from build123d import *

# Parameters (mm, degrees)
SKETCH1_W                                           = 40
SKETCH1_H                                           = 25
BOSS_EXTRUDE1_DEPTH                                 = 10
CUT_EXTRUDE2_REACH                                  = 27.617
SKETCH3_W                                           = 5
SKETCH3_H                                           = 22
F_5_0MM_DOWEL_HOLE1_D                               = 5
CBORE_FOR_M5_HEX_SOCKET_HEAD_CAP_SCREW1_D           = 5.3
CBORE_FOR_M5_HEX_SOCKET_HEAD_CAP_SCREW1_CBORE_D     = 10
CBORE_FOR_M5_HEX_SOCKET_HEAD_CAP_SCREW1_CBORE_DEPTH = 5.4


with BuildPart() as part:
    # Sketch1 → Boss-Extrude1 (new body)
    with BuildSketch(Plane(origin=(0, 0, 0), x_dir=(1, 0, 0), z_dir=(0, 1, 0))):
        Rectangle(SKETCH1_W, SKETCH1_H)
    extrude(amount=BOSS_EXTRUDE1_DEPTH)

    # Sketch3 → Cut-Extrude2 (cut, up to next)
    with BuildSketch(Plane(origin=(0, 10, 0), x_dir=(1, 0, 0), z_dir=(0, 1, 0)), mode=Mode.PRIVATE) as cut_extrude2_sk1:
        with Locations((17.5, -1.5)):
            Rectangle(SKETCH3_W, SKETCH3_H)
    cut_extrude2_tool1 = extrude(cut_extrude2_sk1.sketch, amount=-CUT_EXTRUDE2_REACH, mode=Mode.PRIVATE) & part.part
    add(cut_extrude2_tool1.solids().sort_by_distance((17.5, 10, 1.5))[0], mode=Mode.SUBTRACT)

    # Ø5.0mm Dowel Hole1 (through all)
    with Locations(Plane(origin=(0, 10, 0), x_dir=(1, 0, 0), z_dir=(0, 1, 0))):
        with Locations((-15, 6), (10, -6)):
            Hole(F_5_0MM_DOWEL_HOLE1_D / 2)

    # CBORE for M5 Hex Socket Head Cap Screw1 (through all)
    with Locations(Plane(origin=(0, 10, 0), x_dir=(1, 0, 0), z_dir=(0, 1, 0))):
        with Locations((-12.5, -5), (7.5, 5)):
            CounterBoreHole(CBORE_FOR_M5_HEX_SOCKET_HEAD_CAP_SCREW1_D / 2, CBORE_FOR_M5_HEX_SOCKET_HEAD_CAP_SCREW1_CBORE_D / 2, CBORE_FOR_M5_HEX_SOCKET_HEAD_CAP_SCREW1_CBORE_DEPTH)


solid = part.part
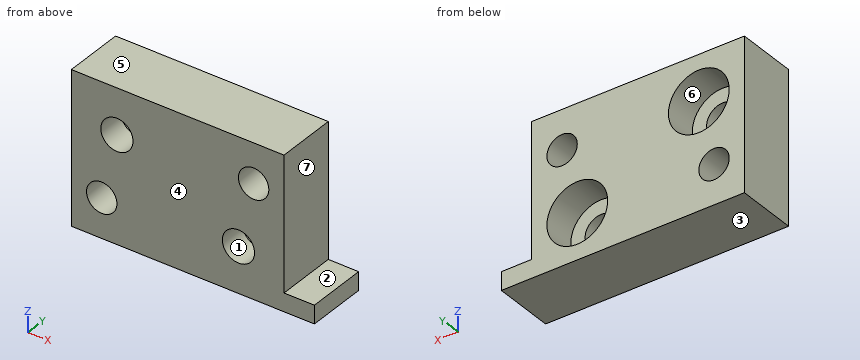
Can you work these out from the model? Positions are in its coordinate system, mm. Face numbers are marked on the shaded views. A direction names the side the tool comes from. Give positions to 0.01 mm unless a question says otherwise; leave off trailing zeros. Order: outer loops, then holes, each group sorted by start corner. A loop starts at its lowest first (then second) coordinate and runs counter-clockwise, first axis right, second up. Notation, with made-up numbers: M 0.5,11.25 L 58.5,11.25 A21 ccw 58.5,45.25 Z; hole C 32,-1 d10. An arc over 180 degrees is marked long. Use a Markdown table: item, result. Add a question column.
Item 1: We'd pull the mould along Z, two halves only. Please class the marked faces 1, 2, 3 and 4: +Z half, -Z half, draft (parallel to the pull), parting line (faces both ways), or undercut.
Item 2: Will these pins go through, and if not, where does the flat tip stop? pin 1 (1 mm diameter, centred on y = 4, z = 9.5, fed in from +X); pin 2 (4.5 mm diameter, centred on x = -15, z = -6, fed in from +Y); pin 3 (11.5 mm diameter, centred on x = 7.5, z = -5, fed in from -Y); pin 4 (4 mm diameter, centred on x = 18.5, y = 3.5, fed in from +Z).
Item 3: Suppose I cut it at C-C (x = 11). List the corners of the cut face in (y, z) for me, then the cut area to 3 significant figures.
Item 4: If I drill on L1, parallel to X at y = 8.25, z = -7; L2, parallel to X at y = 3.5, z = 10; L3, parallel to Y at x = 9, z = -9, over which ranges is the centre line in solid material (lowest first)? Write a range as [from, to].
Item 5: Suppose I cut it at D-D (x = -14.5). List the corners of the cut face in (y, z) for me, then the cut area to 3 significant figures.
Item 6: Suppose I cut it at A-A (y = 7). List the corners of the cut face in (x, z) for me, then the cut area to 3 significant figures.
Item 7: Suppose I cut it at B-B (z = 6). List the corners of the cut face in (x, y) for me.
Item 8: For the marked faces 5, 6 and 7, which set-ups out of +Z, -Z, +X, -X, +Y, -Y let a thin tool reach every point of the face, with its end or its side?
Answer sheet:
| question | item | result |
|---|---|---|
| 1 | face 1 | undercut |
| 1 | face 2 | +Z half |
| 1 | face 3 | -Z half |
| 1 | face 4 | draft |
| 2 | pin 1 | stops at x = 15 |
| 2 | pin 2 | passes through |
| 2 | pin 3 | stops at y = 0 |
| 2 | pin 4 | stops at z = -9.5 |
| 3 | outline | M 0,-12.5 L 10,-12.5 L 10,-8.57 L 4.6,-8.57 L 4.6,-1.43 L 10,-1.43 L 10,3.71 L 0,3.71 Z; M 0,8.29 L 10,8.29 L 10,12.5 L 0,12.5 Z |
| 3 | area | 166 mm² |
| 4 | L1 | x = [-20, -17.29], [-12.71, 2.92], [12.08, 15] |
| 4 | L2 | x = [-20, 15] |
| 4 | L3 | y = [0, 4.6] |
| 5 | outline | M 0,-12.5 L 10,-12.5 L 10,-8.45 L 0,-8.45 Z; M 0,-3.55 L 10,-3.55 L 10,0.42 L 4.6,0.42 L 4.6,3.26 L 0,3.26 Z; M 0,6.74 L 4.6,6.74 L 4.6,9.58 L 10,9.58 L 10,12.5 L 0,12.5 Z |
| 5 | area | 136 mm² |
| 6 | outline | M -20,-12.5 L 20,-12.5 L 20,-9.5 L 15,-9.5 L 15,12.5 L -20,12.5 Z; hole C -15,-6 d5; hole C -12.5,5 d10; hole C 7.5,-5 d10; hole C 10,6 d5 |
| 6 | area | 694 mm² |
| 7 | outline | M -20,0 L -14.95,0 L -14.95,4.6 L -17.4,4.6 L -17.4,10 L -20,10 Z; M -10.05,0 L 7.5,0 L 7.5,10 L -7.6,10 L -7.6,4.6 L -10.05,4.6 Z; M 12.5,0 L 15,0 L 15,10 L 12.5,10 Z |
| 8 | face 5 | +Z, +X, -X, +Y, -Y |
| 8 | face 6 | +Y |
| 8 | face 7 | +Z, +X, +Y, -Y |
